The model under review builds one solid part; all positions refer to its coordinate system, in mm. A direction names the side the tool comes from. Give positions to 0.01 mm unless a question says otherwise; leave off trailing zeros. Order: outer loops, then holes, each group sorted by start corner. A loop starts at its lowest first (then second) coordinate and runs counter-clockwise, first axis right, second up. Notation, with made-up numbers: (-18, -5.5) -> (-7, -5.5) arc R21 ccw to (-7, 12.5) -> close; hole circle Ø3 at (55.25, 2). An arc over 180 degrees is marked (long way). Answer as a JSON object with one key per item and string values. Group by question number.
from build123d import *

# Parameters (mm, degrees)
BOSS_EXTRUDE1_DEPTH = 80
SKETCH4_W           = 60
SKETCH4_H           = 10
CUT_EXTRUDE1_DEPTH  = 90.895772982
SKETCH9_W           = 10
SKETCH9_H           = 5
CUT_EXTRUDE6_DEPTH  = 98.59610648
SKETCH10_W          = 10
SKETCH10_H          = 5
CUT_EXTRUDE7_DEPTH  = 98.59610648
SKETCH12_W          = 5
SKETCH12_H          = 5
CUT_EXTRUDE9_DEPTH  = 98.59610648
SKETCH6_W           = 5
SKETCH6_H           = 5
CUT_EXTRUDE11_DEPTH = 90.895772982


with BuildPart() as part:
    # Sketch1 → Boss-Extrude1 (new body)
    with BuildSketch(Plane.XY):
        Polygon((-7.860697776, 0), (-25.360697776, 0), (-25.360697776, -10), (24.639302224, -10), (24.639302224, 0), (7.139302224, 0), (7.139302224, 25), (-7.860697776, 25), align=None)
    extrude(amount=BOSS_EXTRUDE1_DEPTH)

    # Sketch4 → Cut-Extrude1 (cut, through all)
    with BuildSketch(Plane(origin=(7.139302224, 0, 0), x_dir=(0, 0, -1), z_dir=(1, 0, 0))):
        with Locations((-40, 20)):
            Rectangle(SKETCH4_W, SKETCH4_H)
    extrude(amount=-CUT_EXTRUDE1_DEPTH, mode=Mode.SUBTRACT)

    # Sketch9 → Cut-Extrude6 (cut, through all)
    with BuildSketch(Plane(origin=(24.639302224, 0, 0), x_dir=(0, 0, -1), z_dir=(1, 0, 0))):
        with Locations((-75, -7.5)):
            Rectangle(SKETCH9_W, SKETCH9_H)
    extrude(amount=-CUT_EXTRUDE6_DEPTH, mode=Mode.SUBTRACT)

    # Sketch10 → Cut-Extrude7 (cut, through all)
    with BuildSketch(Plane(origin=(24.639302224, 0, 0), x_dir=(0, 0, -1), z_dir=(1, 0, 0))):
        with Locations((-5, -7.5)):
            Rectangle(SKETCH10_W, SKETCH10_H)
    extrude(amount=-CUT_EXTRUDE7_DEPTH, mode=Mode.SUBTRACT)

    # Sketch12 → Cut-Extrude9 (cut, through all)
    with BuildSketch(Plane(origin=(24.639302224, 0, 0), x_dir=(0, 0, -1), z_dir=(1, 0, 0))):
        with Locations((-39.999750499, -7.5)):
            Rectangle(SKETCH12_W, SKETCH12_H)
    extrude(amount=-CUT_EXTRUDE9_DEPTH, mode=Mode.SUBTRACT)

    # Sketch6 → Cut-Extrude11 (cut, through all)
    with BuildSketch(Plane(origin=(7.139302224, 0, 0), x_dir=(0, 0, -1), z_dir=(1, 0, 0))):
        with Locations((-39.999750499, 12.5)):
            Rectangle(SKETCH6_W, SKETCH6_H)
    extrude(amount=-CUT_EXTRUDE11_DEPTH, mode=Mode.SUBTRACT)


solid = part.part
1. Machinability: for faces 4 (the flat face through (16, 0, 39)), 5 (the flat face through (-16, 0, 39)), 6 (the flat face through (0, -8, 37.5)), 7 (the flat face through (0, -8, 10)), 8 (the flat face through (0, 15, 24)), which of the approach directions +Z, -Z, +X, -X, +Y, -Y give a long, thin tool a straight path to every point of the face, cutting with its end or side? Answer none if there is none.
2. For probe 1 along Z at (x, y) = (-13, -7); probe 2 along Z at (x, y) = (-6.5, 18.5); probe 3 along Y at (x, z) = (1, 64), list the stretches that pass through material, from the lowest coordinate up. Write a range as [from, to].
3. Draft analysis for pull direction Z (two halves, no side actions). For faces 1 (the flat face through (0, 12, 37.5)), 2 (the flat face through (0, -8, 70)), 3 (the flat face through (0, 25, 75)), state which applies: pulls with the +Z half, pulls with the -Z half, needs draft (parallel to the pull), parting line crosses it, or undercut.
4. Take a section at D-D on y = 12. Give the boundary of the cut face in (x, z), plus the area to 4 significant figures.
5. For pin 1 (6 mm diameter, centred on x = -17, z = 8.5, fed in from -Y); pin 2 (4 mm diameter, centred on x = -2.5, z = 39, fed in from +Y); pin 3 (4 mm diameter, centred on x = -14.5, z = 66.5, fed in from +Y); pin 4 (1.5 mm diameter, centred on x = 4.5, y = -7.5, fed in from +Z), all flat-tipped, find the tip position at first contact; note any pin that passes through.
6. Take a section at B-B on z = 22. Give the boundary of the cut face in (x, y), plus the area to 3 significant figures.
7. Take a section at A-A on y = 20. Give the boundary of the cut face in (x, z).
8. Take a section at C-C on x = 9. Give the boundary of the cut face in (y, z), plus the area to 3 significant figures.
Checks:
{
 "1": {"face 4": "+Z, -Z, +X, +Y", "face 5": "+Z, -Z, -X, +Y", "face 6": "+X, -X, -Y", "face 7": "-Z, +X, -X, -Y", "face 8": "+X, -X, +Y"},
 "2": {"probe 1": "z = [10, 37.5], [42.5, 70]", "probe 2": "z = [0, 10], [70, 80]", "probe 3": "y = [-10, 15]"},
 "3": {"face 1": "undercut", "face 2": "pulls with the +Z half", "face 3": "needs draft"},
 "4": {"outline": "(-7.86, 0) -> (7.14, 0) -> (7.14, 37.5) -> (-7.86, 37.5) -> close; (-7.86, 42.5) -> (7.14, 42.5) -> (7.14, 80) -> (-7.86, 80) -> close", "area": "1,125 mm2"},
 "5": {"pin 1": "stops at y = -10", "pin 2": "stops at y = 15", "pin 3": "stops at y = 0", "pin 4": "stops at z = 70"},
 "6": {"outline": "(-25.36, -10) -> (24.64, -10) -> (24.64, 0) -> (7.14, 0) -> (7.14, 15) -> (-7.86, 15) -> (-7.86, 0) -> (-25.36, 0) -> close", "area": "725 mm2"},
 "7": {"outline": "(-7.86, 0) -> (7.14, 0) -> (7.14, 10) -> (-7.86, 10) -> close; (-7.86, 70) -> (7.14, 70) -> (7.14, 80) -> (-7.86, 80) -> close"},
 "8": {"outline": "(-10, 10) -> (-5, 10) -> (-5, 0) -> (0, 0) -> (0, 80) -> (-5, 80) -> (-5, 70) -> (-10, 70) -> (-10, 42.5) -> (-5, 42.5) -> (-5, 37.5) -> (-10, 37.5) -> close", "area": "675 mm2"}
}
